Can you work these out from the drawing? Everything is in mm from the part's minimum corner. Give positions to 0.01 mm unless a question says otherwise; leave off trailing zeros. Write each loop counter-clockwise with the first axis right and the second up, starting at its lowest first coordinate (ties: lowest second). Pieces come first, ordered by that corner, then holes. Notation, with made-up numbers: (-20, 24) - (-15, 24) arc R31 ccw to (-15, 63) - close; hole circle Ø7 at (82, 32.5). An arc over 180 degrees is marked (long way). Write each question's results on one line, items separated by ' | '. Start each with the question number.
Item 1: Suppose I cut it at A-A on x = 11.75. List the corners of the cut face in (y, z) for me.
Item 2: Suppose I cut it at B-B on z = 1.45. List the corners of the cut face in (x, y) for me.
Item 3: We'd pull the mould along Z, two halves only. Please class the marked faces 1, 2 and 3: +Z half, -Z half, draft (parallel to the pull), parting line (faces both ways), or undercut.
Item 4: Will these pins go through, and if not, where does the flat tip stop? P1, Ø1.2, axis at y = 22, z = 1, coming from the +X side; P2, Ø2, axis at x = 10.5, z = 1.5, coming from the +Y side; P3, Ø1.2, axis at x = 10, z = 1.5, coming from the -Y side.
Item 5: Suppose I cut it at C-C on y = 11. List the corners of the cut face in (x, z) for me.
Item 6: Please list where these lines run through material, in increasing order: line 1 along Z through (x, y) = (11.4, 4.25); line 2 along Y through (x, z) = (9.25, 3.75); line 3 along X through (y, z) = (31, 0.4).
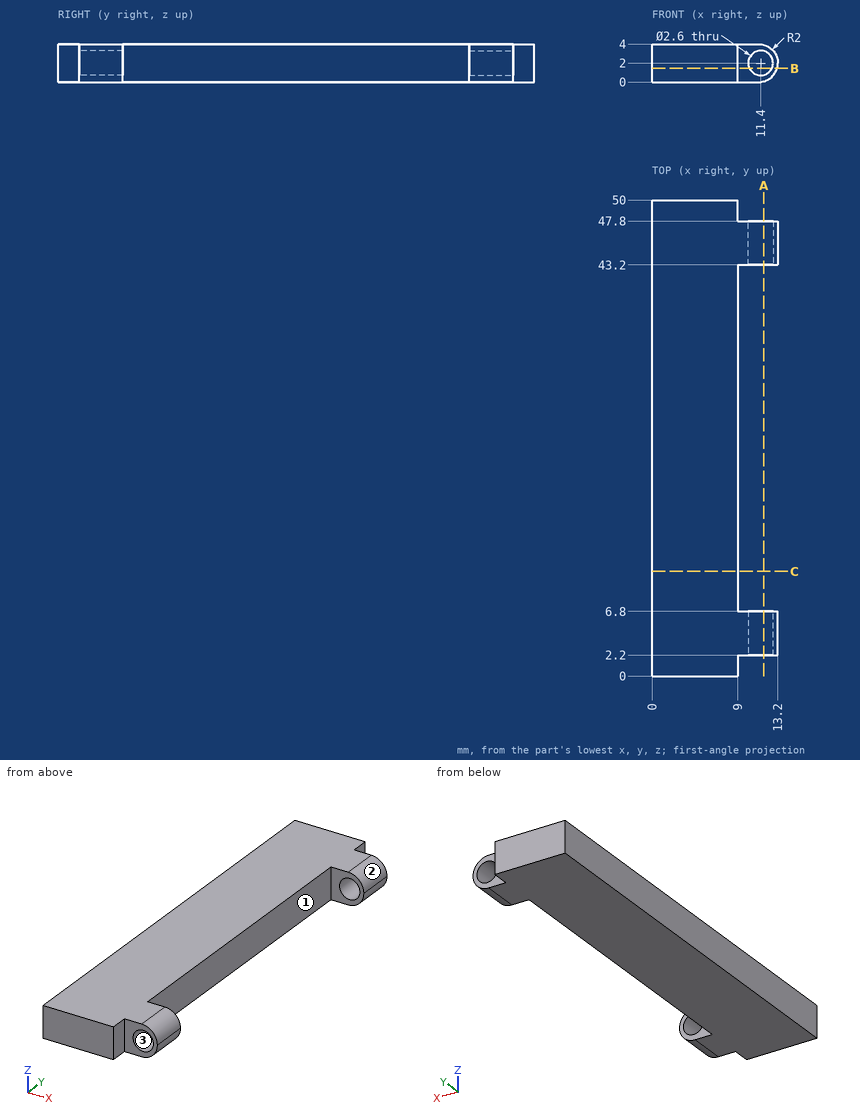
Checked values:
1) outline: (2.2, 0.08) - (6.8, 0.08) - (6.8, 0.75) - (2.2, 0.75) - close; (2.2, 3.25) - (6.8, 3.25) - (6.8, 3.92) - (2.2, 3.92) - close; (43.2, 0.08) - (47.8, 0.08) - (47.8, 0.75) - (43.2, 0.75) - close; (43.2, 3.25) - (47.8, 3.25) - (47.8, 3.92) - (43.2, 3.92) - close
2) outline: (0, 0) - (9, 0) - (9, 2.2) - (10.22, 2.2) - (10.22, 6.8) - (9, 6.8) - (9, 43.2) - (10.22, 43.2) - (10.22, 47.8) - (9, 47.8) - (9, 50) - (0, 50) - close; (12.58, 2.2) - (13.12, 2.2) - (13.12, 6.8) - (12.58, 6.8) - close; (12.58, 43.2) - (13.12, 43.2) - (13.12, 47.8) - (12.58, 47.8) - close
3) face 1: draft | face 2: +Z half | face 3: undercut
4) P1: stops at x = 9 | P2: stops at y = 47.8 | P3: stops at y = 2.2
5) outline: (0, 0) - (9, 0) - (9, 4) - (0, 4) - close
6) line 1: z = 0.01 to 0.7, 3.3 to 3.99 | line 2: y = 2.2 to 6.8, 43.2 to 47.8 | line 3: x = 0 to 9
